Geometry: final body of the model. Coordinates: model frame, mm. Give positions to 0.01 mm unless a question says otherwise; leave off trailing zeros. Loops run counter-clockwise (first coordinate to the right, second up) from the corner with the lowest first, then second, coordinate; pieces in that order, holes last.
```python
from build123d import *

# Parameters (mm, degrees)
F0_W     = 2000
F0_H     = 25
F1_DEPTH = 200
F2_SIZE  = 5
F4_DEPTH = 153
F5_SIZE2 = 15
F5_SIZE  = 20


with BuildPart() as f1:
    # F0 (on Front) → F1 (new body)
    with BuildSketch(Plane.XZ):
        with Locations((-1000, 12.5)):
            Rectangle(F0_W, F0_H)
    extrude(amount=F1_DEPTH)

    # F2
    f2_edges = [f1.edges().sort_by_distance(p)[0] for p in [
        (-1000, -200, 25),
        (-1000, 0, 25),
    ]]
    chamfer(f2_edges, length=F2_SIZE)

    # F3 (on Top) → F4 (cut)
    with BuildSketch(Plane.XY):
        Polygon((0, -200), (0, 0), (-30, 0), align=None)
        Polygon((-2000, 0), (-2000, -200), (-1970, 0), align=None)
    extrude(amount=F4_DEPTH, mode=Mode.SUBTRACT)

    # F5
    f5_edges = [f1.edges().sort_by_distance(p)[0] for p in [
        (-1000, 0, 0),
        (-15, -100, 0),
        (-1985, -100, 0),
    ]]
    f5_side = f1.faces().sort_by_distance((-1000, -100.507614, 0))[0]
    chamfer(f5_edges, length=F5_SIZE, length2=F5_SIZE2, reference=f5_side)


solid = f1.part
```
Q1. Section query A-A, the plane x = -267. Return loops of the section in (y, z), and give its area (4 significant figures).
Q2. Pin query (flat end, axial travel): pin 1 Ø3 at (y, z) = (-33, 19.5) entering from +X (3 decimals); pin 2 Ø3 at (y, z) = (-22, 11) entering from -X; pin 3 Ø1 at (x, z) = (-384, 22.5) entering from +Y. Return the tip coordinate at first contact, or that it passes through.
Q3. Material intervals for probe 1 along X at (y, z) = (-103, 12); probe 2 along Y at (x, z) = (-88, 5.5); probe 3 along X at (y, z) = (-65.5, 11), sorted ascending.
Q4. Section query D-D, the plane y = -36.5. Return loops of the section in (x, z) (3 decimals).
Q5. Section query C-C, the plane z = 10.75. Return loops of the section in (x, y), and give its area (3 significant figures).
Q6. Section query B-B, the plane y = -117.5. Return loops of the section in (x, z) (3 decimals), and give its area (3 significant figures).
Resolved:
1. outline: (-200, 0) - (-20, 0) - (0, 15) - (0, 20) - (-5, 25) - (-195, 25) - (-200, 20) - close
1. area: 4,825 mm2
2. pin 1: stops at x = -24.825
2. pin 2: stops at x = -1969.94
2. pin 3: stops at y = -2
3. probe 1: x = -1981.41 to -18.59
3. probe 2: y = -200 to -12.67
3. probe 3: x = -1974.43 to -25.57
4. outline: (-1975.475, 15) - (-1955.251, 0) - (-44.749, 0) - (-24.525, 15) - (-24.525, 25) - (-1975.475, 25) - close
5. outline: (-1994.27, -200) - (-5.73, -200) - (-34.88, -5.67) - (-1965.12, -5.67) - close
5. area: 381,000 mm2
6. outline: (-1987.625, 15) - (-1967.401, 0) - (-32.599, 0) - (-12.375, 15) - (-12.375, 25) - (-1987.625, 25) - close
6. area: 49,100 mm2
